Autodesk Inventor part; units mm, degrees
ref_plane "YZ Plane" through (0, 0, 0) normal (1, 0, 0) x (0, 1, 0)
ref_plane "XZ Plane" through (0, 0, 0) normal (0, 1, 0) x (-1, 0, 0)
ref_plane "XY Plane" through (0, 0, 0) normal (0, 0, 1) x (1, 0, 0)
sketch "Sketch1" plane through (0, 0, 0) normal (0, 0, 1) x (1, 0, 0)
  line L0 (-8.1893, 41.3629) -> (-15.8199, 41.3629)
  line L1 (-8.1893, 41.3629) -> (0, 18.8629)
  line L2 (-8.1893, 41.3629) -> (26.4246, 41.3629) construction
  line L3 (-4.5496, 31.3629) -> (-19.4596, 31.3629) construction
  line L4 (-12.0046, 31.3629) -> (-12.0046, 41.3629) construction
  line L5 (-15.8199, 41.3629) -> (-24.0093, 18.8629)
  line L6 (-39.5993, 41.3629) -> (-47.2299, 41.3629)
  line L7 (-39.5993, 41.3629) -> (-31.41, 18.8629)
  line L8 (-39.5993, 41.3629) -> (-4.9854, 41.3629) construction
  line L9 (-35.9596, 31.3629) -> (-50.8696, 31.3629) construction
  line L10 (-43.4146, 31.3629) -> (-43.4146, 41.3629) construction
  line L11 (-47.2299, 41.3629) -> (-55.4193, 18.8629)
  line L12 (-71.0093, 41.3629) -> (-78.6399, 41.3629)
  line L13 (-71.0093, 41.3629) -> (-62.82, 18.8629)
  line L14 (-71.0093, 41.3629) -> (-36.3954, 41.3629) construction
  line L15 (-67.3696, 31.3629) -> (-82.2796, 31.3629) construction
  line L16 (-74.8246, 31.3629) -> (-74.8246, 41.3629) construction
  line L17 (-78.6399, 41.3629) -> (-86.8293, 18.8629)
  line L18 (-102.4193, 41.3629) -> (-110.0499, 41.3629)
  line L19 (-102.4193, 41.3629) -> (-94.23, 18.8629)
  line L20 (-102.4193, 41.3629) -> (-67.8054, 41.3629) construction
  line L21 (-98.7796, 31.3629) -> (-113.6896, 31.3629) construction
  line L22 (-106.2346, 31.3629) -> (-106.2346, 41.3629) construction
  line L23 (-110.0499, 41.3629) -> (-118.2393, 18.8629)
  line L24 (-133.8293, 41.3629) -> (-141.4599, 41.3629)
  line L25 (-133.8293, 41.3629) -> (-125.64, 18.8629)
  line L26 (-133.8293, 41.3629) -> (-99.2154, 41.3629) construction
  line L27 (-130.1896, 31.3629) -> (-145.0996, 31.3629) construction
  line L28 (-137.6446, 31.3629) -> (-137.6446, 41.3629) construction
  line L29 (-141.4599, 41.3629) -> (-149.6493, 18.8629)
  line L30 (-165.2393, 41.3629) -> (-172.8699, 41.3629)
  line L31 (-165.2393, 41.3629) -> (-157.05, 18.8629)
  line L32 (-165.2393, 41.3629) -> (-130.6254, 41.3629) construction
  line L33 (-161.5996, 31.3629) -> (-176.5096, 31.3629) construction
  line L34 (-169.0546, 31.3629) -> (-169.0546, 41.3629) construction
  line L35 (-172.8699, 41.3629) -> (-181.0593, 18.8629)
  line L36 (-196.6493, 41.3629) -> (-204.2799, 41.3629)
  line L37 (-196.6493, 41.3629) -> (-188.46, 18.8629)
  line L38 (-196.6493, 41.3629) -> (-162.0354, 41.3629) construction
  line L39 (-193.0096, 31.3629) -> (-207.9196, 31.3629) construction
  line L40 (-200.4646, 31.3629) -> (-200.4646, 41.3629) construction
  line L41 (-204.2799, 41.3629) -> (-212.4693, 18.8629)
  line L42 (-228.0593, 41.3629) -> (-235.6899, 41.3629)
  line L43 (-228.0593, 41.3629) -> (-219.87, 18.8629)
  line L44 (-228.0593, 41.3629) -> (-193.4454, 41.3629) construction
  line L45 (-224.4196, 31.3629) -> (-239.3296, 31.3629) construction
  line L46 (-231.8746, 31.3629) -> (-231.8746, 41.3629) construction
  line L47 (-235.6899, 41.3629) -> (-243.8793, 18.8629)
  line L48 (-259.4693, 41.3629) -> (-267.0999, 41.3629)
  line L49 (-259.4693, 41.3629) -> (-251.28, 18.8629)
  line L50 (-259.4693, 41.3629) -> (-224.8554, 41.3629) construction
  line L51 (-255.8296, 31.3629) -> (-270.7396, 31.3629) construction
  line L52 (-263.2846, 31.3629) -> (-263.2846, 41.3629) construction
  line L53 (-267.0999, 41.3629) -> (-275.2893, 18.8629)
  line L54 (-290.8793, 41.3629) -> (-298.5099, 41.3629)
  line L55 (-290.8793, 41.3629) -> (-282.69, 18.8629)
  line L56 (-290.8793, 41.3629) -> (-256.2654, 41.3629) construction
  line L57 (-287.2396, 31.3629) -> (-302.1496, 31.3629) construction
  line L58 (-294.6946, 31.3629) -> (-294.6946, 41.3629) construction
  line L59 (-298.5099, 41.3629) -> (-306.6993, 18.8629)
  line L60 (-322.2893, 41.3629) -> (-329.9199, 41.3629)
  line L61 (-322.2893, 41.3629) -> (-314.1, 18.8629)
  line L62 (-322.2893, 41.3629) -> (-287.6754, 41.3629) construction
  line L63 (-318.6496, 31.3629) -> (-333.5596, 31.3629) construction
  line L64 (-326.1046, 31.3629) -> (-326.1046, 41.3629) construction
  line L65 (-329.9199, 41.3629) -> (-338.1093, 18.8629)
  line L66 (-353.6993, 41.3629) -> (-361.3299, 41.3629)
  line L67 (-353.6993, 41.3629) -> (-345.51, 18.8629)
  line L68 (-353.6993, 41.3629) -> (-319.0854, 41.3629) construction
  line L69 (-350.0596, 31.3629) -> (-364.9696, 31.3629) construction
  line L70 (-357.5146, 31.3629) -> (-357.5146, 41.3629) construction
  line L71 (-361.3299, 41.3629) -> (-369.5193, 18.8629)
  line L72 (-385.1093, 41.3629) -> (-392.7399, 41.3629)
  line L73 (-385.1093, 41.3629) -> (-376.92, 18.8629)
  line L74 (-385.1093, 41.3629) -> (-350.4954, 41.3629) construction
  line L75 (-381.4696, 31.3629) -> (-396.3796, 31.3629) construction
  line L76 (-388.9246, 31.3629) -> (-388.9246, 41.3629) construction
  line L77 (-392.7399, 41.3629) -> (-400.9293, 18.8629)
  line L78 (-416.5193, 41.3629) -> (-424.1499, 41.3629)
  line L79 (-416.5193, 41.3629) -> (-408.33, 18.8629)
  line L80 (-416.5193, 41.3629) -> (-381.9054, 41.3629) construction
  line L81 (-412.8796, 31.3629) -> (-427.7896, 31.3629) construction
  line L82 (-420.3346, 31.3629) -> (-420.3346, 41.3629) construction
  line L83 (-424.1499, 41.3629) -> (-432.3393, 18.8629)
  line L84 (-447.9293, 41.3629) -> (-455.5599, 41.3629)
  line L85 (-447.9293, 41.3629) -> (-439.74, 18.8629)
  line L86 (-447.9293, 41.3629) -> (-413.3154, 41.3629) construction
  line L87 (-444.2896, 31.3629) -> (-459.1996, 31.3629) construction
  line L88 (-451.7446, 31.3629) -> (-451.7446, 41.3629) construction
  line L89 (-455.5599, 41.3629) -> (-463.7493, 18.8629)
  line L90 (-479.3393, 41.3629) -> (-486.9699, 41.3629)
  line L91 (-479.3393, 41.3629) -> (-471.15, 18.8629)
  line L92 (-479.3393, 41.3629) -> (-444.7254, 41.3629) construction
  line L93 (-475.6996, 31.3629) -> (-490.6096, 31.3629) construction
  line L94 (-483.1546, 31.3629) -> (-483.1546, 41.3629) construction
  line L95 (-486.9699, 41.3629) -> (-495.1593, 18.8629)
  line L96 (-510.7493, 41.3629) -> (-518.3799, 41.3629)
  line L97 (-510.7493, 41.3629) -> (-502.56, 18.8629)
  line L98 (-510.7493, 41.3629) -> (-476.1354, 41.3629) construction
  line L99 (-507.1096, 31.3629) -> (-522.0196, 31.3629) construction
  line L100 (-514.5646, 31.3629) -> (-514.5646, 41.3629) construction
  line L101 (-518.3799, 41.3629) -> (-526.5693, 18.8629)
  line L102 (-542.1593, 41.3629) -> (-549.7899, 41.3629)
  line L103 (-542.1593, 41.3629) -> (-533.97, 18.8629)
  line L104 (-542.1593, 41.3629) -> (-507.5454, 41.3629) construction
  line L105 (-538.5196, 31.3629) -> (-553.4296, 31.3629) construction
  line L106 (-545.9746, 31.3629) -> (-545.9746, 41.3629) construction
  line L107 (-549.7899, 41.3629) -> (-557.9793, 18.8629)
  line L108 (-573.5693, 41.3629) -> (-581.1999, 41.3629)
  line L109 (-573.5693, 41.3629) -> (-565.38, 18.8629)
  line L110 (-573.5693, 41.3629) -> (-538.9554, 41.3629) construction
  line L111 (-569.9296, 31.3629) -> (-584.8396, 31.3629) construction
  line L112 (-577.3846, 31.3629) -> (-577.3846, 41.3629) construction
  line L113 (-581.1999, 41.3629) -> (-589.3893, 18.8629)
  line L114 (-604.9793, 41.3629) -> (-612.6099, 41.3629)
  line L115 (-604.9793, 41.3629) -> (-596.79, 18.8629)
  line L116 (-604.9793, 41.3629) -> (-570.3654, 41.3629) construction
  line L117 (-601.3396, 31.3629) -> (-616.2496, 31.3629) construction
  line L118 (-608.7946, 31.3629) -> (-608.7946, 41.3629) construction
  line L119 (-612.6099, 41.3629) -> (-620.7993, 18.8629)
  line L120 (-620.7993, 18.8629) -> (-620.7993, 0)
  line L121 (-620.7993, 0) -> (0, 0)
  line L122 (0, 0) -> (0, 18.8629)
  line L123 (-24.0093, 18.8629) -> (-31.41, 18.8629)
  line L124 (-55.4193, 18.8629) -> (-62.82, 18.8629)
  line L125 (-86.8293, 18.8629) -> (-94.23, 18.8629)
  line L126 (-118.2393, 18.8629) -> (-125.64, 18.8629)
  line L127 (-149.6493, 18.8629) -> (-157.05, 18.8629)
  line L128 (-181.0593, 18.8629) -> (-188.46, 18.8629)
  line L129 (-212.4693, 18.8629) -> (-219.87, 18.8629)
  line L130 (-243.8793, 18.8629) -> (-251.28, 18.8629)
  line L131 (-275.2893, 18.8629) -> (-282.69, 18.8629)
  line L132 (-306.6993, 18.8629) -> (-314.1, 18.8629)
  line L133 (-338.1093, 18.8629) -> (-345.51, 18.8629)
  line L134 (-369.5193, 18.8629) -> (-376.92, 18.8629)
  line L135 (-400.9293, 18.8629) -> (-408.33, 18.8629)
  line L136 (-432.3393, 18.8629) -> (-439.74, 18.8629)
  line L137 (-463.7493, 18.8629) -> (-471.15, 18.8629)
  line L138 (-495.1593, 18.8629) -> (-502.56, 18.8629)
  line L139 (-526.5693, 18.8629) -> (-533.97, 18.8629)
  line L140 (-557.9793, 18.8629) -> (-565.38, 18.8629)
  line L141 (-589.3893, 18.8629) -> (-596.79, 18.8629)
  point P0 (2.0713, 13.1721)
  point P1 (-26.0805, 13.1721)
  point P2 (-29.3387, 13.1721)
  point P3 (-57.4905, 13.1721)
  point P4 (-60.7487, 13.1721)
  point P5 (-88.9005, 13.1721)
  point P6 (-92.1587, 13.1721)
  point P7 (-120.3105, 13.1721)
  point P8 (-123.5687, 13.1721)
  point P9 (-151.7205, 13.1721)
  point P10 (-154.9787, 13.1721)
  point P11 (-183.1305, 13.1721)
  point P12 (-186.3887, 13.1721)
  point P13 (-214.5405, 13.1721)
  point P14 (-217.7987, 13.1721)
  point P15 (-245.9505, 13.1721)
  point P16 (-249.2087, 13.1721)
  point P17 (-277.3605, 13.1721)
  point P18 (-280.6187, 13.1721)
  point P19 (-308.7705, 13.1721)
  point P20 (-312.0287, 13.1721)
  point P21 (-340.1805, 13.1721)
  point P22 (-343.4387, 13.1721)
  point P23 (-371.5905, 13.1721)
  point P24 (-374.8487, 13.1721)
  point P25 (-403.0005, 13.1721)
  point P26 (-406.2587, 13.1721)
  point P27 (-434.4105, 13.1721)
  point P28 (-437.6687, 13.1721)
  point P29 (-465.8205, 13.1721)
  point P30 (-469.0787, 13.1721)
  point P31 (-497.2305, 13.1721)
  point P32 (-500.4887, 13.1721)
  point P33 (-528.6405, 13.1721)
  point P34 (-531.8987, 13.1721)
  point P35 (-560.0505, 13.1721)
  point P36 (-563.3087, 13.1721)
  point P37 (-591.4605, 13.1721)
  point P38 (-594.7187, 13.1721)
  point P39 (-622.8705, 13.1721)
  point P40 (-59.1196, 18.8629)
  point P41 (0, 9.4315)
  dimension "d3" = 30
  dimension "d4" = 70
  dimension "d5" = 14.91
  dimension "d8" = 31.41
  dimension "d14" = 620.7993
  dimension "d15" = 18.8629
  dimension "d16" = 18.8629
  dimension "d18" = 13.1722
  dimension "d19" = 13.1722
  dimension "d20" = 24.0093
  dimension "d21" = 22.5
  dimension "d22" = 23.944
  dimension "d23" = 3.0107
  dimension "d24" = 18.8629
extrude "Extrusion1" add sketch "Sketch1" along normal mid plane 20
sketch "Sketch2" plane through (0, 0, 0) normal (0, 1, 0) x (-1, 0, 0)
  line L0 (8.1893, -10) -> (8.1893, 10) construction
  line L1 (0, 10) -> (8.1893, 10) construction
  line L2 (0, -10) -> (0, 10) construction
  line L3 (8.1893, -10) -> (0, -10) construction
  line L4 (0, -10) -> (-15, -10)
  line L5 (-15, -10) -> (-15, 10)
  line L6 (-15, 10) -> (0, 10)
  line L7 (0, 10) -> (0, -10)
  line L8 (620.7993, -10) -> (620.7993, 10) construction
  line L9 (612.6099, 10) -> (620.7993, 10) construction
  line L10 (612.6099, 10) -> (612.6099, -10) construction
  line L11 (620.7993, -10) -> (612.6099, -10) construction
  line L12 (620.7993, -10) -> (635.7993, -10)
  line L13 (635.7993, -10) -> (635.7993, 10)
  line L14 (635.7993, 10) -> (620.7993, 10)
  line L15 (620.7993, 10) -> (620.7993, -10)
  point P0 (0, 0)
  dimension "d27" = 15
  dimension "d28" = 20
  dimension "d29" = 15
  dimension "d30" = 20
extrude "Extrusion2" add sketch "Sketch2" along normal blind 10
sketch "Sketch3" plane through (0, 10, 0) normal (0, 1, 0) x (1, 0, 0)
  line L0 (0, -10) -> (15, -10) construction
  line L1 (15, -10) -> (15, 10) construction
  line L2 (15, 10) -> (0, 10) construction
  line L3 (0, -10) -> (0, 10) construction
  line L4 (-635.7993, 10) -> (-635.7993, -10) construction
  line L5 (-635.7993, -10) -> (-620.7993, -10) construction
  line L6 (-620.7993, 10) -> (-620.7993, -10) construction
  line L7 (-620.7993, 10) -> (-635.7993, 10) construction
  line L8 (15, 10) -> (-635.7993, 10) construction
  line L9 (-635.7993, -10) -> (15, -10) construction
  line L10 (-310.3996, -10) -> (-310.3996, 10) construction
  circle A0 centre (7.5, 0) radius 2.65
  circle A1 centre (-628.2993, 0) radius 2.65
  point P0 (0, 0)
  point P1 (0, -12.5)
  point P2 (-620.7993, -12.5)
  point P3 (0, 0)
  point P4 (7.5, 10)
  dimension "d33" = 5.3
extrude "Extrusion3" cut sketch "Sketch3" against normal through all
sketch "Sketch4" plane through (0, 10, 0) normal (0, 1, 0) x (1, 0, 0)
  circle A0 centre (-628.2993, 0) radius 2.65 construction
  line L0 (-635.7993, 10) -> (-635.7993, -10) construction
  line L1 (-635.7993, -10) -> (-620.7993, -10) construction
  line L2 (-620.7993, 10) -> (-620.7993, -10) construction
  line L3 (-620.7993, 10) -> (-635.7993, 10) construction
  circle A1 centre (7.5, 0) radius 2.65 construction
  line L4 (0, -10) -> (15, -10) construction
  line L5 (15, -10) -> (15, 10) construction
  line L6 (15, 10) -> (0, 10) construction
  line L7 (0, -10) -> (0, 10) construction
  line L8 (15, 10) -> (-635.7993, 10) construction
  line L9 (-635.7993, -10) -> (15, -10) construction
  line L10 (-310.3996, 10) -> (-310.3996, -10) construction
  circle A2 centre (7.5, 0) radius 4.35
  circle A3 centre (-628.2993, 0) radius 4.35
  point P0 (0, 0)
  point P1 (-620.7993, -12.5)
  point P2 (0, -12.5)
  dimension "d36" = 8.7
extrude "Extrusion4" cut sketch "Sketch4" against normal blind 3.5
properties part number "cremallera1"
The model under review builds one solid part; all positions refer to its coordinate system, in mm. A direction names the side the tool comes from. Give positions to 0.01 mm unless a question says otherwise; leave off trailing zeros. Use one line per item in the form item = value. Start each with the question number.
Item 1: For faces 1 (the flat face through (8, 10, 5)), 2 (the flat face through (-349.66, 30.27, -0.14)), 3 (the flat face through (-616.647, 30.27, -0.14)), list the 3-axis set-ups (+Z, -Z, +X, -X, +Y, -Y) from which the entire face can be reached by the end or side of a thin tool; tool diameter is ignored.
Item 2: Insertion check: pin 1 Ø3.5 at (x, z) = (-309.5, 2) entering from +Y; pin 2 Ø1 at (y, z) = (22.5, 3.5) entering from +X; pin 3 Ø9.5 at (y, z) = (16, -2.5) entering from +X. Each pin has a flat end and moves straight along its axis. Give the tip position at first contact, or say it passes through.
Item 3: To check wall thickness, follow line 1 along X through (y, z) = (8.7, 0); line 2 along X through (y, z) = (1.75, 0); line 3 along Z through (x, y) = (7, 3). State the ranges of each line that lie inside material, in increasing order. Write a range as from..to.
Item 4: The part is to be moulded in two halves that separate along X. For faces 4 (the flat face through (-365.367, 30.27, -0.14)), 5 (the flat face through (-315, 0, 0)), 6 (the flat face through (-635.799, 5, 0)), say which applies: pulls with the +X half, pulls with the -X half, needs draft (parallel to the pull), parting line crosses it, or undercut.
Completed:
q1.face_1 = +Z, -Z, +X, +Y
q1.face_2 = +Z, -Z, +Y
q1.face_3 = +Z, -Z, -X, +Y
q2.pin_1 = 18.86
q2.pin_2 = -1.14
q2.pin_3 = 0
q3.line_1 = -635.8..-632.65, -623.95..3.15, 11.85..15
q3.line_2 = -635.8..-630.95, -625.65..4.85, 10.15..15
q3.line_3 = -10..-2.6, 2.6..10
q4.face_4 = undercut
q4.face_5 = needs draft
q4.face_6 = pulls with the -X half
